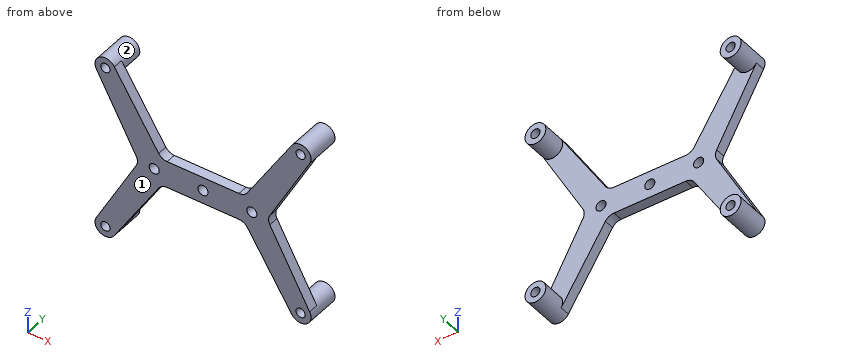
```python
from build123d import *

# Parameters (mm, degrees)
SKETCH1_R           = 1.5
SKETCH1_R_2         = 4
SKETCH1_R_3         = 3.1
SKETCH1_R_4         = 1.375
BOSS_EXTRUDE1_DEPTH = 3
SKETCH2_R           = 3.1
SKETCH2_R_2         = 1.375
BOSS_EXTRUDE2_DEPTH = 7
FILLET4_R           = 3


with BuildPart() as part:
    # Sketch1 → Boss-Extrude1 (new body)
    with BuildSketch(Plane(origin=(0, 0, 0), x_dir=(1, 0, 0), z_dir=(0, 1, 0))):
        with BuildLine():
            ThreePointArc((10.93588599, 22.68421055), (10.5, 24.5), (10.93588599, 26.31578945))
            Line((10.93588599, 26.31578945), (9.937320588, 24.5))
            Line((9.937320588, 24.5), (10.93588599, 22.68421055))
        make_face()
        with BuildLine():
            Line((16.695320866, 28.5), (14.5, 28.5))
            ThreePointArc((14.5, 28.5), (16.370485645, 28.035715409), (17.806752459, 26.750641726))
            Line((17.806752459, 26.750641726), (16.695320866, 28.5))
        make_face()
        with BuildLine():
            Line((14.5, 20.5), (16.695320866, 20.5))
            Line((16.695320866, 20.5), (17.806752459, 22.249358274))
            ThreePointArc((17.806752459, 22.249358274), (16.370485645, 20.964284591), (14.5, 20.5))
        make_face()
        with BuildLine():
            ThreePointArc((17.806752459, 26.750641726), (16.370485645, 28.035715409), (14.5, 28.5))
            ThreePointArc((14.5, 28.5), (12.518729486, 27.974847788), (11.057693269, 26.537283576))
            Line((11.057693269, 26.537283576), (10.93588599, 26.31578945))
            ThreePointArc((10.93588599, 26.31578945), (10.5, 24.5), (10.93588599, 22.68421055))
            Line((10.93588599, 22.68421055), (11.057693269, 22.462716424))
            ThreePointArc((11.057693269, 22.462716424), (12.518729486, 21.025152212), (14.5, 20.5))
            ThreePointArc((14.5, 20.5), (16.370485645, 20.964284591), (17.806752459, 22.249358274))
            Line((17.806752459, 22.249358274), (17.942306731, 22.462716424))
            ThreePointArc((17.942306731, 22.462716424), (18.35805825, 23.443881381), (18.5, 24.5))
            ThreePointArc((18.5, 24.5), (18.35805825, 25.556118619), (17.942306731, 26.537283576))
            Line((17.942306731, 26.537283576), (17.806752459, 26.750641726))
        make_face()
        with Locations((14.5, 24.5)):
            Circle(SKETCH1_R, mode=Mode.SUBTRACT)
        with BuildLine():
            Line((29, 28.5), (16.695320866, 28.5))
            Line((16.695320866, 28.5), (17.806752459, 26.750641726))
            ThreePointArc((17.806752459, 26.750641726), (17.876215398, 26.645033703), (17.942306731, 26.537283576))
            ThreePointArc((17.942306731, 26.537283576), (18.35805825, 25.556118619), (18.5, 24.5))
            ThreePointArc((18.5, 24.5), (18.35805825, 23.443881381), (17.942306731, 22.462716424))
            ThreePointArc((17.942306731, 22.462716424), (17.876215398, 22.354966297), (17.806752459, 22.249358274))
            Line((17.806752459, 22.249358274), (16.695320866, 20.5))
            Line((16.695320866, 20.5), (29, 20.5))
            ThreePointArc((29, 20.5), (25, 24.5), (29, 28.5))
        make_face()
        with Locations((29, 24.5)):
            Circle(SKETCH1_R_2)
        with Locations((29, 24.5)):
            Circle(SKETCH1_R, mode=Mode.SUBTRACT)
        with BuildLine():
            Line((41.304679134, 28.5), (29, 28.5))
            ThreePointArc((29, 28.5), (31.828427125, 27.328427125), (33, 24.5))
            ThreePointArc((33, 24.5), (31.828427125, 21.671572875), (29, 20.5))
            Line((29, 20.5), (41.304679134, 20.5))
            Line((41.304679134, 20.5), (40.193247541, 22.249358274))
            ThreePointArc((40.193247541, 22.249358274), (40.123784602, 22.354966297), (40.057693269, 22.462716424))
            ThreePointArc((40.057693269, 22.462716424), (39.5, 24.5), (40.057693269, 26.537283576))
            ThreePointArc((40.057693269, 26.537283576), (40.123784602, 26.645033703), (40.193247541, 26.750641726))
            Line((40.193247541, 26.750641726), (41.304679134, 28.5))
        make_face()
        with BuildLine():
            Line((40.193247541, 22.249358274), (41.304679134, 20.5))
            Line((41.304679134, 20.5), (43.5, 20.5))
            ThreePointArc((43.5, 20.5), (41.629514355, 20.964284591), (40.193247541, 22.249358274))
        make_face()
        with BuildLine():
            Line((43.5, 28.5), (41.304679134, 28.5))
            Line((41.304679134, 28.5), (40.193247541, 26.750641726))
            ThreePointArc((40.193247541, 26.750641726), (41.629514355, 28.035715409), (43.5, 28.5))
        make_face()
        with BuildLine():
            Line((48.062679412, 24.5), (47.06411401, 26.31578945))
            ThreePointArc((47.06411401, 26.31578945), (47.389502284, 25.433687303), (47.5, 24.5))
            ThreePointArc((47.5, 24.5), (47.389502284, 23.566312697), (47.06411401, 22.68421055))
            Line((47.06411401, 22.68421055), (48.062679412, 24.5))
        make_face()
        with BuildLine():
            ThreePointArc((46.942306731, 26.537283576), (45.481270514, 27.974847788), (43.5, 28.5))
            ThreePointArc((43.5, 28.5), (41.629514355, 28.035715409), (40.193247541, 26.750641726))
            Line((40.193247541, 26.750641726), (40.057693269, 26.537283576))
            ThreePointArc((40.057693269, 26.537283576), (39.5, 24.5), (40.057693269, 22.462716424))
            Line((40.057693269, 22.462716424), (40.193247541, 22.249358274))
            ThreePointArc((40.193247541, 22.249358274), (41.629514355, 20.964284591), (43.5, 20.5))
            ThreePointArc((43.5, 20.5), (45.481270514, 21.025152212), (46.942306731, 22.462716424))
            Line((46.942306731, 22.462716424), (47.06411401, 22.68421055))
            ThreePointArc((47.06411401, 22.68421055), (47.389502284, 23.566312697), (47.5, 24.5))
            ThreePointArc((47.5, 24.5), (47.389502284, 25.433687303), (47.06411401, 26.31578945))
            Line((47.06411401, 26.31578945), (46.942306731, 26.537283576))
        make_face()
        with Locations((43.5, 24.5)):
            Circle(SKETCH1_R, mode=Mode.SUBTRACT)
        with BuildLine():
            Line((43.5, 20.5), (41.304679134, 20.5))
            Line((41.304679134, 20.5), (55.332212283, -1.578894771))
            ThreePointArc((55.332212283, -1.578894771), (56.421105229, 2.667787717), (60.667787717, 1.578894771))
            Line((60.667787717, 1.578894771), (48.062679412, 24.5))
            Line((48.062679412, 24.5), (47.06411401, 22.68421055))
            ThreePointArc((47.06411401, 22.68421055), (47.004960458, 22.572501054), (46.942306731, 22.462716424))
            ThreePointArc((46.942306731, 22.462716424), (45.481270514, 21.025152212), (43.5, 20.5))
        make_face()
        with BuildLine():
            Line((55.332212283, 50.578894771), (41.304679134, 28.5))
            Line((41.304679134, 28.5), (43.5, 28.5))
            ThreePointArc((43.5, 28.5), (45.481270514, 27.974847788), (46.942306731, 26.537283576))
            ThreePointArc((46.942306731, 26.537283576), (47.004960458, 26.427498946), (47.06411401, 26.31578945))
            Line((47.06411401, 26.31578945), (48.062679412, 24.5))
            Line((48.062679412, 24.5), (60.667787717, 47.421105229))
            ThreePointArc((60.667787717, 47.421105229), (56.421105229, 46.332212283), (55.332212283, 50.578894771))
        make_face()
        with BuildLine():
            Line((10.93588599, 22.68421055), (9.937320588, 24.5))
            Line((9.937320588, 24.5), (-2.667787717, 1.578894771))
            ThreePointArc((-2.667787717, 1.578894771), (0.81849193, 2.989995144), (3.1, 0))
            ThreePointArc((3.1, 0), (2.989995144, -0.81849193), (2.667787717, -1.578894771))
            Line((2.667787717, -1.578894771), (16.695320866, 20.5))
            Line((16.695320866, 20.5), (14.5, 20.5))
            ThreePointArc((14.5, 20.5), (12.518729486, 21.025152212), (11.057693269, 22.462716424))
            ThreePointArc((11.057693269, 22.462716424), (10.995039542, 22.572501054), (10.93588599, 22.68421055))
        make_face()
        Circle(SKETCH1_R_3)
        Circle(SKETCH1_R_4, mode=Mode.SUBTRACT)
        with Locations((0, 49)):
            Circle(SKETCH1_R_3)
        with Locations((0, 49)):
            Circle(SKETCH1_R_4, mode=Mode.SUBTRACT)
        with BuildLine():
            ThreePointArc((11.057693269, 26.537283576), (12.518729486, 27.974847788), (14.5, 28.5))
            Line((14.5, 28.5), (16.695320866, 28.5))
            Line((16.695320866, 28.5), (2.667787717, 50.578894771))
            ThreePointArc((2.667787717, 50.578894771), (2.989995144, 49.81849193), (3.1, 49))
            ThreePointArc((3.1, 49), (0.81849193, 46.010004856), (-2.667787717, 47.421105229))
            Line((-2.667787717, 47.421105229), (9.937320588, 24.5))
            Line((9.937320588, 24.5), (10.93588599, 26.31578945))
            ThreePointArc((10.93588599, 26.31578945), (10.995039542, 26.427498946), (11.057693269, 26.537283576))
        make_face()
        with Locations((58, 49)):
            Circle(SKETCH1_R_3)
        with Locations((58, 49)):
            Circle(SKETCH1_R_4, mode=Mode.SUBTRACT)
        with Locations((58, 0)):
            Circle(SKETCH1_R_3)
        with Locations((58, 0)):
            Circle(SKETCH1_R_4, mode=Mode.SUBTRACT)
    extrude(amount=BOSS_EXTRUDE1_DEPTH)

    # Sketch2 → Boss-Extrude2 (add)
    with BuildSketch(Plane(origin=(0, 3, 0), x_dir=(1, 0, 0), z_dir=(0, 1, 0))):
        with Locations((0, 49)):
            Circle(SKETCH2_R)
        with Locations((0, 49)):
            Circle(SKETCH2_R_2, mode=Mode.SUBTRACT)
        with Locations((58, 49)):
            Circle(SKETCH2_R)
        with Locations((58, 49)):
            Circle(SKETCH2_R_2, mode=Mode.SUBTRACT)
        with Locations((58, 0)):
            Circle(SKETCH2_R)
        with Locations((58, 0)):
            Circle(SKETCH2_R_2, mode=Mode.SUBTRACT)
        Circle(SKETCH2_R)
        Circle(SKETCH2_R_2, mode=Mode.SUBTRACT)
    extrude(amount=BOSS_EXTRUDE2_DEPTH)

    # Fillet4
    fillet4_edges = [part.edges().sort_by_distance(p)[0] for p in [
        (41.304679134, 1.5, -20.5),
        (16.695320866, 1.5, -20.5),
        (9.937320588, 1.5, -24.5),
        (16.695320866, 1.5, -28.5),
        (41.304679134, 1.5, -28.5),
        (48.062679412, 1.5, -24.5),
    ]]
    fillet(fillet4_edges, radius=FILLET4_R)


solid = part.part
```
For this review, take the finished solid that the model builds, in its own axes (mm). Face numbers are marked on the shaded views. A direction names the side the tool comes from. Give positions to 0.01 mm unless a question says otherwise; leave off trailing zeros. Write each loop counter-clockwise with the first axis right and the second up, starting at its lowest first coordinate (ties: lowest second). Pieces come first, ordered by that corner, then holes. Notation, with made-up numbers: M 32.5,-26.75 L 89.5,-26.75 A37 ccw 89.5,12.25 Z; hole C 65,-25.75 d8. An arc over 180 degrees is marked long. One line per item, written item: value.
1) Take a section at C-C, the plane z = -24.5. Write out the cut boundary in (x, y).
Results are:
outline: M 9.51,0 L 13,0 L 13,3 L 9.51,3 Z; M 16,0 L 27.5,0 L 27.5,3 L 16,3 Z; M 30.5,0 L 42,0 L 42,3 L 30.5,3 Z; M 45,0 L 48.49,0 L 48.49,3 L 45,3 Z
2) Take a section at B-B, the plane x = 0. Write out the cut boundary in (y, z) (3 decimals).
Results are:
outline: M 0,-52.1 L 10,-52.1 L 10,-50.375 L 0,-50.375 Z; M 0,-47.625 L 10,-47.625 L 10,-45.9 L 3,-45.9 L 3,-42.57 L 0,-42.57 Z; M 0,-6.43 L 3,-6.43 L 3,-3.1 L 10,-3.1 L 10,-1.375 L 0,-1.375 Z; M 0,1.375 L 10,1.375 L 10,3.1 L 0,3.1 Z
3) For the marked faces 1 and 2, list the 3-axis set-ups (+Z, -Z, +X, -X, +Y, -Y) from which the entire face can be reached by the end or side of a thin tool; tool diameter is ignored.
Results are:
face 1: +Z, -Z, +X, -X, -Y
face 2: +Y
4) Take a section at A-A, the plane y = 7. Write out the cut boundary in (x, z) (3 decimals), then the cut area to 3 significant figures.
Results are:
outline: C 0,-49 d6.2; C 0,0 d6.2; C 58,-49 d6.2; C 58,0 d6.2; hole C 0,-49 d2.75; hole C 0,0 d2.75; hole C 58,-49 d2.75; hole C 58,0 d2.75
area: 97.0 mm²
5) For P1, Ø5, axis at x = 20.5, z = -19, coming from the +Y side; P2, Ø2.5, axis at x = 31, y = 2, coming from the -Z side; P3, Ø0.9, axis at x = 26, y = 2, coming from the +Z side, all flat-tipped, find the tip position at first contact; note any pin that passes through.
Results are:
P1: stops at y = 3
P2: stops at z = -28.5
P3: stops at z = -20.5
6) For line 1 (Z direction, x = 58, y = 8) (3 decimals); line 2 (X direction, y = 4, z = -49) (3 decimals); line 3 (X direction, y = 2.75, z = -49) (3 decimals), list the stretches that pass through material, from the lowest coordinate up. Write a range as from..to.
Results are:
line 1: z = -52.1..-50.375, -47.625..-45.9, -3.1..-1.375, 1.375..3.1
line 2: x = -3.1..-1.375, 1.375..3.1, 54.9..56.625, 59.375..61.1
line 3: x = -3.1..-1.375, 1.375..3.671, 54.329..56.625, 59.375..61.1
7) Take a section at D-D, the plane x = 29. Write out the cut boundary in (y, z).
Results are:
outline: M 0,-28.5 L 3,-28.5 L 3,-26 L 0,-26 Z; M 0,-23 L 3,-23 L 3,-20.5 L 0,-20.5 Z
